Print and shaded views of the part. All mm, measured from the part's lowest x, y and z. A direction names the side the tool comes from. Coordinates: 2 decimals unless noted, no trailing zeros. Order: outer loops, then holes, each group sorted by start corner. A loop starts at its lowest first (then second) coordinate and runs counter-clockwise, first axis right, second up.
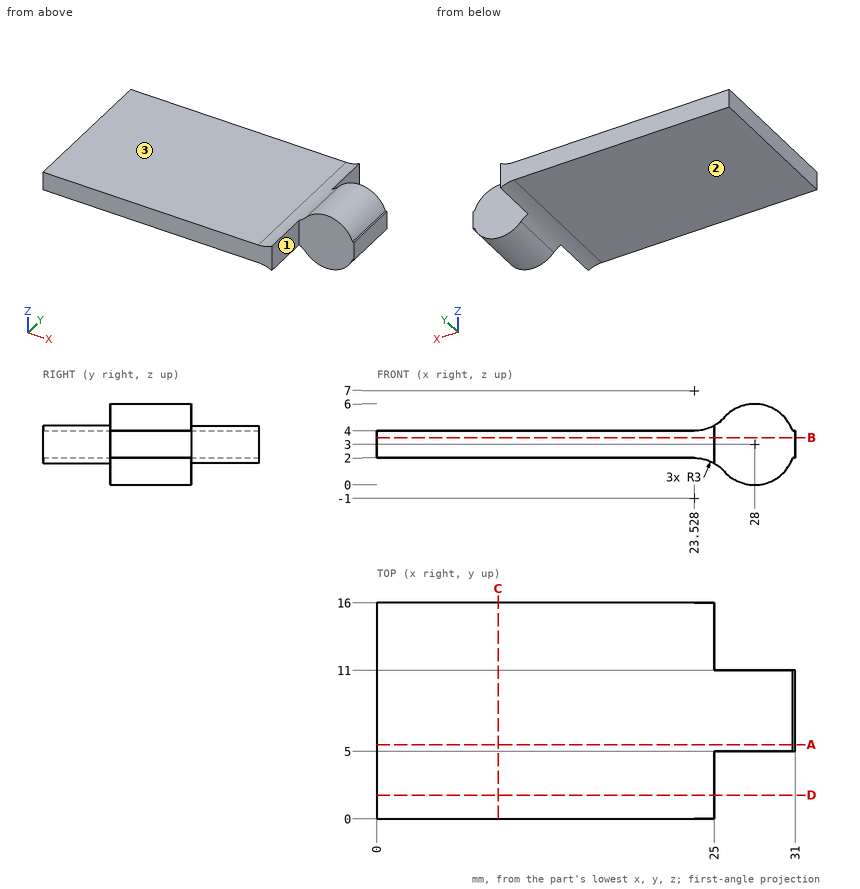
Q1. Drop flat-ended pins along their axis: P1, Ø4, axis at x = 5, y = 14, coming from the +Z side; P2, Ø8, axis at x = 8.5, y = 7, coming from the -Z side; P3, Ø3, axis at y = 2.5, z = 4, coming from the +X side. Give the stop position or say it passes through.
Established:
P1: stops at z = 4
P2: stops at z = 2
P3: stops at x = 25
Q2. Cut at D-D, the plane y = 1.75. List the corners of the cut face in (x, z), plus the area to 3 significant figures.
Established:
outline: (0, 2) - (23.53, 2) arc R3 cw to (25, 1.61) - (25, 4.39) arc R3 cw to (23.53, 4) - (0, 4) - close
area: 50.4 mm2
Q3. Which spindle directions (+Z, -Z, +X, -X, +Y, -Y) get a long thin tool onto all of the face, cutting with end or side? Do the marked faces 1, 2 and 3. Say none if no direction does.
Established:
face 1: +Z, -Z, +X, -Y
face 2: -Z, -X, +Y, -Y
face 3: +Z, -X, +Y, -Y
Q4. Cut at C-C, the plane x = 9. List the corners of the cut face in (y, z), plus the area to 3 significant figures.
Established:
outline: (0, 2) - (16, 2) - (16, 4) - (0, 4) - close
area: 32.0 mm2
Q5. Cut at B-B, the plane z = 3.5. List the corners of the cut face in (x, y).
Established:
outline: (0, 0) - (25, 0) - (25, 5) - (31, 5) - (31, 11) - (25, 11) - (25, 16) - (0, 16) - close
Q6. Cut at A-A, the plane y = 5.5. List the corners of the cut face in (x, z), plus the area to 3 significant figures.
Established:
outline: (0, 2) - (23.53, 2) arc R3 cw to (25.76, 1) arc R3 ccw to (30.83, 2) - (31, 2) - (31, 4) - (30.83, 4) arc R3 ccw to (25.76, 5) arc R3 cw to (23.53, 4) - (0, 4) - close
area: 79.2 mm2
Q7. Probe line 1 (Y direction, x = 28, z = 4.75); line 2 (Z direction, x = 7, y = 6); line 3 (X direction, y = 3, z = 3.8). List the from-to ranges inside material, lowest first.
Established:
line 1: y = 5 to 11
line 2: z = 2 to 4
line 3: x = 0 to 25
